For this review, take the finished solid that the model builds, in its own axes (mm). Give positions to 0.01 mm unless a question says otherwise; leave off trailing zeros. Order: outer loops, then holes, each group sorted by start corner. A loop starts at its lowest first (then second) coordinate and runs counter-clockwise, first axis right, second up.
from build123d import *

# Parameters (mm, degrees)
SKETCH1_R             = 11
BOSS_EXTRUDE1_DEPTH   = 655
BOSS_EXTRUDE1_2_DEPTH = 655
SKETCH2_W             = 426
SKETCH2_H             = 40
BOSS_EXTRUDE2_DEPTH   = 2
LPATTERN1_COUNT       = 2
LPATTERN1_PITCH       = 570
SKETCH3_R             = 3.5
CUT_EXTRUDE1_DEPTH    = 22
SKETCH4_R             = 3.5
CUT_EXTRUDE2_DEPTH    = 22


with BuildPart() as part:
    # Sketch1 → Boss-Extrude1 (new body)
    with BuildSketch(Plane.XY):
        with Locations((-219, 0)):
            Circle(SKETCH1_R)
    extrude(amount=BOSS_EXTRUDE1_DEPTH)



with BuildPart() as body_2:
    # Sketch1 → Boss-Extrude1 2 (new body)
    with BuildSketch(Plane.XY):
        with Locations((219, 0)):
            Circle(SKETCH1_R)
    extrude(amount=BOSS_EXTRUDE1_2_DEPTH)


with BuildPart() as part_1:
    add(part.part)

    add(body_2.part)  # Boss-Extrude2 merges body 2
    # Sketch2 → Boss-Extrude2 (add)
    with BuildSketch(Plane(origin=(0, 8, 0), x_dir=(1, 0, 0), z_dir=(0, 1, 0))):
        with Locations((0, -23)):
            Rectangle(SKETCH2_W, SKETCH2_H)
    boss_extrude2 = extrude(amount=BOSS_EXTRUDE2_DEPTH)

    # LPattern1: Boss-Extrude2 ×2
    with Locations(*[(0, 0, i * LPATTERN1_PITCH) for i in range(1, LPATTERN1_COUNT)]):
        add(boss_extrude2)

    # Sketch3 → Cut-Extrude1 (cut, through all)
    with BuildSketch(Plane(origin=(0, 10, 0), x_dir=(1, 0, 0), z_dir=(0, 1, 0))):
        with Locations((-193.5, -35)):
            Circle(SKETCH3_R)
        with Locations((193.5, -35)):
            Circle(SKETCH3_R)
    extrude(amount=-CUT_EXTRUDE1_DEPTH, mode=Mode.SUBTRACT)

    # Sketch4 → Cut-Extrude2 (cut, through all)
    with BuildSketch(Plane(origin=(0, 10, 0), x_dir=(1, 0, 0), z_dir=(0, 1, 0))):
        with Locations((-193.5, -605)):
            Circle(SKETCH4_R)
        with Locations((193.5, -605)):
            Circle(SKETCH4_R)
    extrude(amount=-CUT_EXTRUDE2_DEPTH, mode=Mode.SUBTRACT)


solid = part_1.part
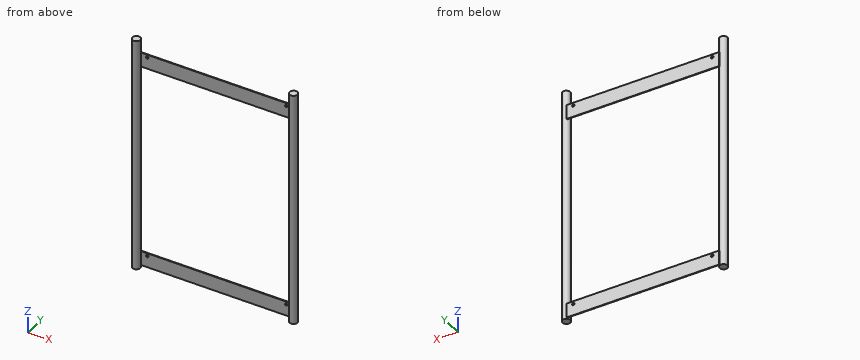
1) We need section D-D on z = 172.5. Give the boundary of the cut face in (x, y), then the cut area to 3 significant figures.
Answer sheet:
outline: circle Ø22 at (-219, 0); circle Ø22 at (219, 0)
area: 760 mm2
2) To check wall thickness, follow line 1 (Z direction, x = -193.5, y = 8.65); line 2 (X direction, y = 9.1, z = 605); line 3 (X direction, y = 8.8, z = 35). State the ranges of each line that lie inside material, in increasing order.
Answer sheet:
line 1: z = 3 to 31.5, 38.5 to 43, 573 to 601.5, 608.5 to 613
line 2: x = -225.18 to -197, -190 to 190, 197 to 225.18
line 3: x = -225.6 to -197, -190 to 190, 197 to 225.6
3) We need section C-C on z = 594. Give the boundary of the cut face in (x, y), then the cut area to 3 significant figures.
Answer sheet:
outline: (-213, 9.22) arc R11 ccw (long way) to (-211.45, 8) - (211.45, 8) arc R11 ccw (long way) to (213, 9.22) - (213, 10) - (-213, 10) - close
area: 1,610 mm2
4) Clearance check with flat-ended pins moving along their axes: pin 1 (10 mm diameter, centred on y = -7.5, z = 189, fed in from +X); pin 2 (1 mm diameter, centred on x = -44, y = 8.5, fed in from +Z); pin 3 (0.6 mm diameter, centred on y = 9.5, z = 30.5, fed in from +X). State where each tip first meets the part, or that it passes through.
Answer sheet:
pin 1: stops at x = 229.71
pin 2: stops at z = 613
pin 3: stops at x = 225.03
5) We need section A-A on x = 143. Give the boundary of the cut face in (y, z).
Answer sheet:
outline: (8, 3) - (10, 3) - (10, 43) - (8, 43) - close; (8, 573) - (10, 573) - (10, 613) - (8, 613) - close
6) We need section B-B on y = -7.25. Give the boundary of the cut face in (x, z), then the cut area to 3 significant figures.
Answer sheet:
outline: (-227.27, 0) - (-210.73, 0) - (-210.73, 655) - (-227.27, 655) - close; (210.73, 0) - (227.27, 0) - (227.27, 655) - (210.73, 655) - close
area: 21,700 mm2
